Build history of the part. All positions in model axes, mm. Face numbers are marked on the shaded views. A direction names the side the tool comes from. Round coordinates to 2 decimals unless told otherwise and drop trailing zeros. Loops run counter-clockwise (first coordinate to the right, second up) from the corner with the lowest first, then second, coordinate; pieces in that order, holes last. Notation, with made-up numbers: (-28.75, -16.5) - (15.25, -16.5) arc R23 ccw to (15.25, 1.5) - close; hole circle Ø4 at (17.5, 19.5). An arc over 180 degrees is marked (long way). Use a Markdown table: item, result.
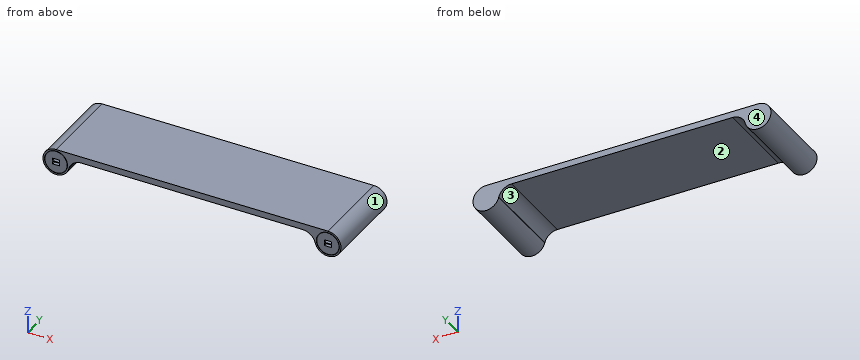
from build123d import *

# Parameters (mm, degrees)
F1_DEPTH = 160
F2_R     = 22
F2_R_2   = 21.25
F3_DEPTH = 0.5
F4_W     = 13
F4_H     = 5
F5_DEPTH = 15


with BuildPart() as f1:
    # F0 (on Front) → F1 (new body)
    with BuildSketch(Plane.XZ):
        with BuildLine():
            Line((235.599727, 19.470476), (235.851854, 18.529524))
            ThreePointArc((235.851854, 18.529524), (279.833834, 9.780964), (260, 50))
            Line((260, 50), (0, 50))
            Line((0, 50), (-260, 50))
            ThreePointArc((-260, 50), (-279.833834, 9.780964), (-235.851854, 18.529524))
            Line((-235.851854, 18.529524), (-235.599727, 19.470476))
            ThreePointArc((-235.599727, 19.470476), (-226.670617, 32.833834), (-211.451581, 38))
            Line((-211.451581, 38), (0, 38))
            Line((0, 38), (211.451581, 38))
            ThreePointArc((211.451581, 38), (226.670617, 32.833834), (235.599727, 19.470476))
        make_face()
    extrude(amount=-F1_DEPTH)

    # F2 (on face) → F3 (cut)
    with BuildSketch(Plane.XZ):
        with Locations((260, 25)):
            Circle(F2_R)
        with Locations((260, 25)):
            Circle(F2_R_2, mode=Mode.SUBTRACT)
        with Locations((-260, 25)):
            Circle(F2_R)
        with Locations((-260, 25)):
            Circle(F2_R_2, mode=Mode.SUBTRACT)
    extrude(amount=-F3_DEPTH, mode=Mode.SUBTRACT)

    # F4 (on face) → F5 (cut)
    with BuildSketch(Plane.XZ):
        with Locations((260, 28.25)):
            Rectangle(F4_W, F4_H)
        with Locations((260, 21.75)):
            Rectangle(F4_W, F4_H)
        with Locations((-260, 28.25)):
            Rectangle(F4_W, F4_H)
        with Locations((-260, 21.75)):
            Rectangle(F4_W, F4_H)
    extrude(amount=-F5_DEPTH, mode=Mode.SUBTRACT)


solid = f1.part
Q1. Drop flat-ended pins along their axis: pin 1 (8 mm diameter, centred on y = 48, z = 6, fed in from +X); pin 2 (1.5 mm diameter, centred on y = 8.5, z = 21.5, fed in from -X); pin 3 (8 mm diameter, centred on x = 157, y = 129.5, fed in from -Z); pin 4 (12 mm diameter, centred on x = -95, z = 28.5, fed in from +Y). Give the stop position or say it passes through.
Results found:
| item | result |
|---|---|
| pin 1 | stops at x = 280 |
| pin 2 | stops at x = -284.85 |
| pin 3 | stops at z = 38 |
| pin 4 | passes through |
Q2. Cut at B-B, the plane y = 105.5. List the corners of the cut face in (x, z).
Results found:
| item | result |
|---|---|
| outline | (-260, 50) arc R25 ccw (long way) to (-235.85, 18.53) - (-235.6, 19.47) arc R25 cw to (-211.45, 38) - (211.45, 38) arc R25 cw to (235.6, 19.47) - (235.85, 18.53) arc R25 ccw (long way) to (260, 50) - close |
Q3. Cut at A-A, the plane z = 9.5. List the corners of the cut face in (x, y), plus the area to 3 significant figures.
Results found:
| item | result |
|---|---|
| outline | (-279.62, 0) - (-275.61, 0) - (-275.61, 0.5) - (-274.54, 0.5) - (-274.54, 0) - (-245.46, 0) - (-245.46, 0.5) - (-244.39, 0.5) - (-244.39, 0) - (-240.38, 0) - (-240.38, 160) - (-279.62, 160) - close; (240.38, 0) - (244.39, 0) - (244.39, 0.5) - (245.46, 0.5) - (245.46, 0) - (274.54, 0) - (274.54, 0.5) - (275.61, 0.5) - (275.61, 0) - (279.62, 0) - (279.62, 160) - (240.38, 160) - close |
| area | 12,600 mm2 |
Q4. Cut at C-C, the plane x = -180. List the corners of the cut face in (y, z), plus the area to 3 significant figures.
Results found:
| item | result |
|---|---|
| outline | (0, 38) - (160, 38) - (160, 50) - (0, 50) - close |
| area | 1,920 mm2 |
Q5. Which spindle directions (+Z, -Z, +X, -X, +Y, -Y) get a long thin tool onto all of the face, cutting with end or side? Do the marked faces 1 and 2. Say none if no direction does.
Results found:
| item | result |
|---|---|
| face 1 | +Y, -Y |
| face 2 | -Z, +Y, -Y |
Q6. Pull direction X, two halves, no side cores. Call the marked faces 3 and 4: pulls with the +X half, pulls with the -X half, needs draft (parallel to the pull), parting line crosses it, or undercut.
Results found:
| item | result |
|---|---|
| face 3 | undercut |
| face 4 | needs draft |
Q7. Probe line 1 (Z direction, x = -260, y = 0.45); line 2 (Z direction, x = 65.5, y = 91); line 3 (X direction, y = 146.5, z = 27). List the from-to ranges inside material, lowest first.
Results found:
| item | result |
|---|---|
| line 1 | z = 0 to 3, 3.75 to 19.25, 24.25 to 25.75, 30.75 to 46.25, 47 to 50 |
| line 2 | z = 38 to 50 |
| line 3 | x = -284.92 to -232.16, 232.16 to 284.92 |
